For this review, take the finished solid that the model builds, in its own axes (mm). Face numbers are marked on the shaded views. Give positions to 0.01 mm unless a question says otherwise; leave off trailing zeros. Order: outer loops, then holes, each group sorted by start corner. A loop starts at its lowest first (then second) coordinate and runs counter-clockwise, first axis right, second up. Notation, with made-up numbers: M -31.75,16.5 L -22.75,16.5 A18 cw -22.75,46.5 Z; hole C -29,13 d1. An arc over 180 degrees is marked long. Answer as CSV lines item,"result". Start each with the question number.
1. Mouldability with a two-part tool opening along Y and no side actions: class the marked faces 1, 2 and 3 as pulls with the +Y half, pulls with the -Y half, needs draft (parallel to the pull), parting line crosses it, or undercut.
2. Clearance check with flat-ended pins moving along their axes: P1, Ø4, axis at y = -11, z = -14, coming from the -X side; P2, Ø8, axis at y = -4, z = -40.5, coming from the -X side; P3, Ø8, axis at y = -20.5, z = -31.5, coming from the +X side. State where each tip first meets the part, or that it passes through.
3. For line 1 along Y through (x, z) = (-37, -38); line 2 along X through (y, z) = (-11.5, -19); line 3 along Z through (x, y) = (-21.5, -18.25), list the stretches that pass through material, from the lowest coordinate up.
4. We need section B-B, the plane x = -18.5. Give the boundary of the cut face in (y, z).
5. We need section D-D, the plane x = -11. Give the boundary of the cut face in (y, z), and give its area (3 significant figures).
6. We need section C-C, the plane y = -4.75. Give the boundary of the cut face in (x, z), and give its area (3 significant figures).
7. We need section A-A, the plane y = -13.75. Give the boundary of the cut face in (x, z).
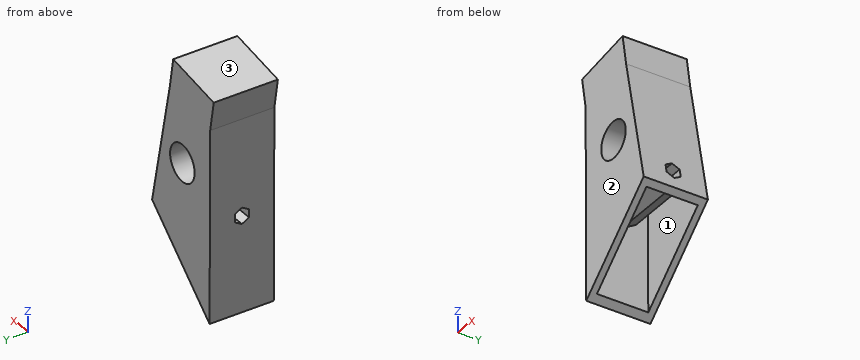
from build123d import *

# Parameters (mm, degrees)
F2_DEPTH = 25
F1_R     = 7.15
F3_DEPTH = 25.4
F6_DEPTH = 35.2
F7_T     = -2.5
F8_DEPTH = 12


with BuildPart() as f2:
    # F0 (on Front) → F2 (new body)
    with BuildSketch(Plane.XZ):
        Polygon((-15.0582233108, 4.0902668196), (-38.706164358, 0.000163102), (-38.330538716, -74.8110767319), (-4.764814752, -44.8387198881), align=None)
    extrude(amount=F2_DEPTH)

    # F1 (on Front) → F3 (cut)
    with BuildSketch(Plane.XZ):
        with Locations((-22.4353701932, -21.2910585503)):
            Circle(F1_R)
    extrude(amount=F3_DEPTH, mode=Mode.SUBTRACT)

    # F5 (on face) → F6 (cut, symmetric)
    with BuildSketch(Plane(origin=(-38.7051877725, 0, -0.1943379235), x_dir=(0, -1, 0), z_dir=(-0.9999873951, 0, -0.0050209154))):
        Polygon((15.2337295342, -35.6725638611), (12.4837295342, -34.0848506209), (9.7337295342, -35.6725638611), (9.7337295342, -38.8479903417), (12.4837295342, -40.435703582), (15.2337295342, -38.8479903417), align=None)
    extrude(amount=F6_DEPTH, both=True, mode=Mode.SUBTRACT)

    # F7
    f7_openings = [f2.faces().sort_by_distance(p)[0] for p in [
        (-21.547677, -12.5, -59.824898),
    ]]
    offset(amount=F7_T, openings=f7_openings, kind=Kind.INTERSECTION)

    # F8 (add): a face of the model
    f8_faces = [f2.faces().sort_by_distance(p)[0] for p in [
        (-26.8821938344, -12.5, 2.0452149608),
    ]]
    extrude(f8_faces, amount=F8_DEPTH)


solid = f2.part
Result set:
1,face 1,"undercut"
1,face 2,"pulls with the -Y half"
1,face 3,"needs draft"
2,P1,"x = -38.65"
2,P2,"x = -38.52"
2,P3,"x = -6.73"
3,line 1,"-25 to -15.23, -9.73 to 0"
3,line 2,"-38.61 to -36.11, -31.81 to -29.21, -15.66 to -13.06, -12.76 to -10.2"
3,line 3,"-30.9 to -28.38, -14.2 to -11.69, 0.44 to 15.15"
4,outline,"M -25,-57.1 L -22.5,-57.1 L -22.5,-30.1 L -2.5,-30.1 L -2.5,-57.1 L 0,-57.1 L 0,-27.26 L -25,-27.26 Z; M -25,-15.32 L 0,-15.32 L 0,15.67 L -25,15.67 Z; M -17.73,-40.38 L -12.48,-43.42 L -7.23,-40.38 L -7.23,-34.32 L -12.48,-31.29 L -17.73,-34.32 Z; hole M -22.5,-12.48 L -2.5,-12.48 L -2.5,0.96 L -22.5,0.96 Z; hole M -15.23,-38.94 L -12.48,-40.53 L -9.73,-38.94 L -9.73,-35.77 L -12.48,-34.18 L -15.23,-35.77 Z"
5,outline,"M -25,-50.41 L -22.5,-50.41 L -22.5,-27.34 L -2.5,-27.34 L -2.5,-50.41 L 0,-50.41 L 0,-15.2 L -25,-15.2 Z; M -17.73,-40.35 L -12.48,-43.38 L -7.23,-40.35 L -7.23,-34.28 L -12.48,-31.25 L -17.73,-34.28 Z; hole M -15.23,-38.9 L -12.48,-40.49 L -9.73,-38.9 L -9.73,-35.73 L -12.48,-34.14 L -15.23,-35.73 Z"
5,area,"488 mm2"
6,outline,"M -40.75,11.82 L -38.71,0 L -38.33,-74.81 L -35.84,-72.59 L -36.2,-2.1 L -17.01,1.22 L -6.92,-46.76 L -4.76,-44.84 L -15.06,4.09 L -17.1,15.91 Z; C -22.44,-21.29 d19.3; hole C -22.44,-21.29 d14.3"
6,area,"780 mm2"
7,outline,"M -40.75,11.82 L -38.71,0 L -38.53,-35.01 L -6.87,-34.85 L -15.06,4.09 L -17.1,15.91 Z; M -38.51,-39.9 L -38.33,-74.81 L -35.84,-72.59 L -35.99,-42.77 L -7.78,-42.63 L -6.92,-46.76 L -4.76,-44.84 L -5.84,-39.73 Z; C -22.44,-21.29 d19.3; hole M -36.2,-2.1 L -36.04,-32.11 L -10.02,-31.98 L -17.01,1.22 Z; hole C -22.44,-21.29 d14.3"
